Part print with two shaded views. Sizes in mm from the minimum x, y, z corner. A direction names the side the tool comes from. Give positions to 0.01 mm unless a question says otherwise; leave off trailing zeros. Write each loop counter-clockwise with the first axis right and the second up, starting at its lowest first coordinate (ties: lowest second). Pieces come first, ordered by that corner, then holes.
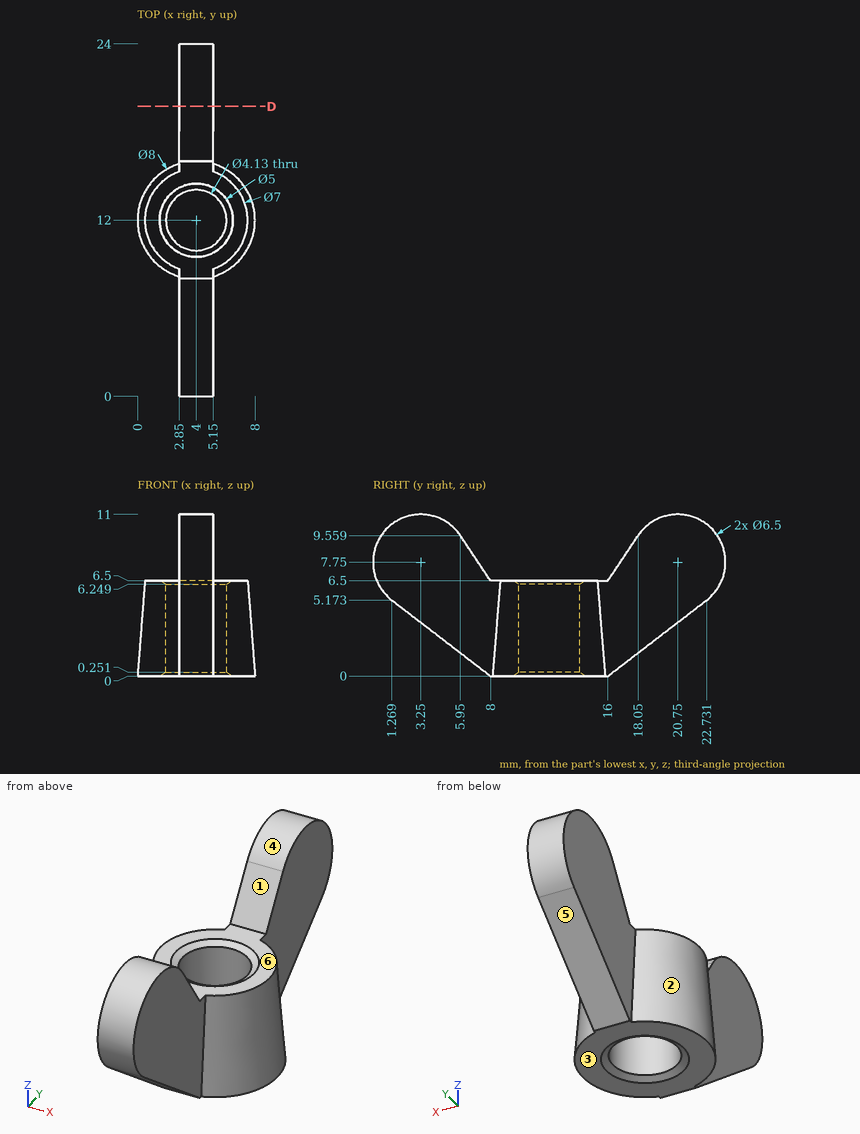
1) Drill centre lines: L1, parallel to X at y = 12, z = 2.2 (1 decimal); L2, parallel to Y at x = 3.75, z = 10 (1 decimal); L3, parallel to Y at x = 4, z = 4.05 (1 decimal). Where is each one in solid material? Low to high.
Check result:
L1: x = 0.2 to 1.9, 6.1 to 7.8
L2: y = 0.9 to 5.6, 18.4 to 23.1
L3: y = 2.7 to 9.9, 14.1 to 21.3
2) 3-axis set-ups, long thin cutter, end or side, ignore diameter. For the marked faces 5 and 6: which of +Z, -Z, +X, -X, +Y, -Y reach the whole face in a straight line?
Check result:
face 5: -Z, +X, -X, +Y
face 6: +Z, +X, -X
3) Flat gauge pins, fed straight in: P1, Ø5, axis at y = 19.5, z = 3.5, coming from the -X side; P2, Ø3.5, axis at x = 4.5, y = 11.5, coming from the +Z side (1 decimal); P3, Ø1.5, axis at y = 14, z = 6, coming from the -X side; P4, Ø1, axis at y = 12.5, z = 8.5, coming from the +X side. Where does each tip first touch, or does it go through?
Check result:
P1: stops at x = 2.85
P2: stops at z = 6.5
P3: stops at x = 0.68
P4: passes through
4) Saw through at D-D (y = 19.75). Write the cut outline in (x, z), and give its area (3 significant figures).
Check result:
outline: (2.85, 2.88) - (5.15, 2.88) - (5.15, 10.84) - (2.85, 10.84) - close
area: 18.3 mm2
5) Mould opens along Y. For the marked faces 1, 2, 3 and 4 say: +Y half, -Y half, draft (parallel to the pull), parting line (faces both ways), or undercut.
Check result:
face 1: undercut
face 2: parting line
face 3: draft
face 4: undercut
